Part print with two shaded views. Sizes in mm from the minimum x, y, z corner. A direction names the side the tool comes from. Round coordinates to 2 decimals unless told otherwise and drop trailing zeros. Order: outer loops, then holes, each group sorted by start corner. A loop starts at its lowest first (then second) coordinate and runs counter-clockwise, first axis right, second up. Notation, with made-up numbers: M -11,-38 L 24,-38 A11 cw 24,-31 Z; hole C 57.5,-10 d3. An arc over 180 degrees is marked long. Put each result on its own line as item: value.
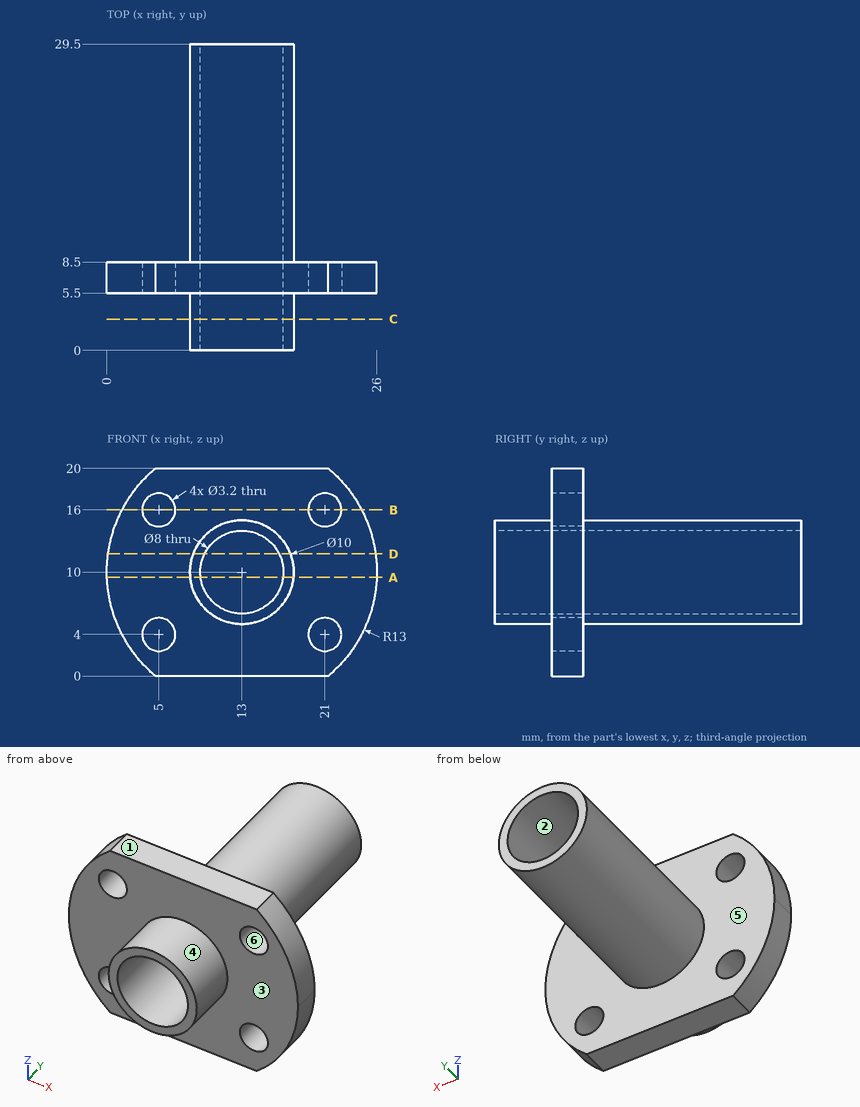
Item 1: Probe line 1 along X through (y, z) = (6.35, 4); line 2 along X through (y, z) = (10, 10); line 3 along Y through (x, z) = (16.5, 16.5). List the from-to ranges inside material, lowest first. Write a range as [from, to].
Answers below:
line 1: [1.47, 3.4], [6.6, 19.4], [22.6, 24.53]
line 2: [8, 9], [17, 18]
line 3: [5.5, 8.5]
Item 2: Mould opens along Z. For the marked faces 1, 2 and 3 say: pulls with the +Z half, pulls with the -Z half, needs draft (parallel to the pull), parting line crosses it, or undercut.
Answers below:
face 1: pulls with the +Z half
face 2: undercut
face 3: needs draft
Item 3: Band-saw the part on D-D on z = 11.75. Give the cut face in (x, y).
Answers below:
outline: M 0.12,5.5 L 8.32,5.5 L 8.32,0 L 9.4,0 L 9.4,29.5 L 8.32,29.5 L 8.32,8.5 L 0.12,8.5 Z; M 16.6,0 L 17.68,0 L 17.68,5.5 L 25.88,5.5 L 25.88,8.5 L 17.68,8.5 L 17.68,29.5 L 16.6,29.5 Z
Item 4: Pin check, flat tips, straight feed: P1, Ø3.5, axis at x = 21, z = 4, coming from the +Y side; P2, Ø1.5, axis at x = 6, y = 5, coming from the +Z side; P3, Ø10, axis at y = 19.5, z = 15.5, coming from the +X side; P4, Ø6, axis at x = 6, y = 21, coming from the +Z side. Stop position of each tip, or through.
Answers below:
P1: y = 8.5
P2: z = 20
P3: x = 17.97
P4: z = 13
Item 5: Band-saw the part on A-A on z = 9.5. Give the cut face in (x, y).
Answers below:
outline: M 0.01,5.5 L 8.03,5.5 L 8.03,0 L 9.03,0 L 9.03,29.5 L 8.03,29.5 L 8.03,8.5 L 0.01,8.5 Z; M 16.97,0 L 17.97,0 L 17.97,5.5 L 25.99,5.5 L 25.99,8.5 L 17.97,8.5 L 17.97,29.5 L 16.97,29.5 Z
Item 6: Band-saw the part on B-B on z = 16. Give the cut face in (x, y), and give its area (3 significant figures).
Answers below:
outline: M 1.47,5.5 L 3.4,5.5 L 3.4,8.5 L 1.47,8.5 Z; M 6.6,5.5 L 19.4,5.5 L 19.4,8.5 L 6.6,8.5 Z; M 22.6,5.5 L 24.53,5.5 L 24.53,8.5 L 22.6,8.5 Z
area: 50.0 mm²
Item 7: Tool access for the marked faces 4, 5 and 6: list every direction of +Z, -Z, +X, -X, +Y, -Y with a clear straight run to the whole face (end or side of a thin tool).
Answers below:
face 4: -Y
face 5: +Y
face 6: +Y, -Y
Item 8: Band-saw the part on C-C on y = 3. Give the cut face in (x, z).
Answers below:
outline: C 13,10 d10; hole C 13,10 d8
